The listing builds one solid part. Answer for the finished solid, in the listing's coordinates (mm). A direction names the side the tool comes from. Give positions to 0.01 mm unless a question says otherwise; leave off trailing zeros. Loops run counter-clockwise (first coordinate to the right, second up) from the corner with the lowest first, then second, coordinate; pieces in that order, holes last. Notation, with made-up numbers: (-4.75, 26) - (45.25, 26) arc R33 ccw to (45.25, 58) - close; hole circle Ø5 at (73.25, 60.25). An arc over 180 degrees is marked (long way). Write each question's results on one line, items separated by ' | '.
from build123d import *

# Parameters (mm, degrees)
SKETCH1_W           = 25.4
SKETCH1_H           = 25.4
SKETCH1_W_2         = 23
SKETCH1_H_2         = 23
BOSS_EXTRUDE1_DEPTH = 115
CUT_EXTRUDE1_START  = -24.2
SKETCH2_W           = 40.231781255
SKETCH2_H           = 27.281754711
CUT_EXTRUDE1_DEPTH  = 24.2
SKETCH5_R           = 1
SKETCH5_R_2         = 2.5
SKETCH5_R_3         = 1.25
CUT_EXTRUDE4_DEPTH  = 10
CUT_EXTRUDE2_REACH  = 142.365
SKETCH3_R           = 1.25
SKETCH3_R_2         = 1.05
SKETCH3_R_3         = 2.5
SKETCH6_R           = 1.6
SKETCH6_R_2         = 1.25
CUT_EXTRUDE5_DEPTH  = 8
SKETCH3_3_R         = 1.25
CUT_EXTRUDE9_DEPTH  = 141.364864582
SKETCH10_R          = 1.55
SKETCH10_R_2        = 1.25
SKETCH10_W          = 7.208576747
SKETCH10_H          = 12.490715562
SKETCH10_W_2        = 3.851256807
SKETCH10_H_2        = 11.057621271
CUT_EXTRUDE10_DEPTH = 5
FILLET1_R           = 3.5
SKETCH11_R          = 1.25
CUT_EXTRUDE11_DEPTH = 8


with BuildPart() as part:
    # Sketch1 → Boss-Extrude1 (new body)
    with BuildSketch(Plane.XY):
        with Locations((63.668417616, 21.669583611)):
            Rectangle(SKETCH1_W, SKETCH1_H)
        with Locations((63.668417616, 21.669583611)):
            Rectangle(SKETCH1_W_2, SKETCH1_H_2, mode=Mode.SUBTRACT)
    extrude(amount=BOSS_EXTRUDE1_DEPTH)

    # Sketch2 → Cut-Extrude1 (cut)
    with BuildSketch(Plane.ZY.offset(-50.968417616).offset(CUT_EXTRUDE1_START)):
        with Locations((94.884109373, 23.810460967)):
            Rectangle(SKETCH2_W, SKETCH2_H)
    extrude(amount=CUT_EXTRUDE1_DEPTH, mode=Mode.SUBTRACT)

    # Sketch5 → Cut-Extrude4 (cut)
    with BuildSketch(Plane(origin=(76.368417616, 0, 0), x_dir=(0, 0, -1), z_dir=(1, 0, 0))):
        with Locations((-102.757359313, 25.912224298)):
            Circle(SKETCH5_R)
        with Locations((-111.242640687, 25.912224298)):
            Circle(SKETCH5_R)
        with Locations((-111.242640687, 17.426942923)):
            Circle(SKETCH5_R)
        with Locations((-102.757359313, 17.426942923)):
            Circle(SKETCH5_R)
        with Locations((-107, 21.669583611)):
            Circle(SKETCH5_R_2)
        with Locations((-16.95, 29.737819564)):
            Circle(SKETCH5_R_3)
        with Locations((-75, 29.737819564)):
            Circle(SKETCH5_R_3)
        with Locations((-19.204163056, 23.117794927)):
            Circle(SKETCH5_R_3)
        with BuildLine():
            Line((-95.356264863, 19.604734734), (-95.356264863, 24.520728377))
            ThreePointArc((-95.356264863, 24.520728377), (-94.114846786, 25.762146454), (-92.87342871, 24.520728377))
            Line((-92.87342871, 24.520728377), (-92.87342871, 19.604734734))
            ThreePointArc((-92.87342871, 19.604734734), (-94.114846786, 18.363316658), (-95.356264863, 19.604734734))
        make_face()
    extrude(amount=-CUT_EXTRUDE4_DEPTH, mode=Mode.SUBTRACT)

    # Sketch3 → Cut-Extrude2 (cut, up to next)
    with BuildSketch(Plane.XZ.offset(-8.969583611), mode=Mode.PRIVATE) as cut_extrude2_sk1:
        with Locations(Location((54.918417616, 32, 0), (0, 0, 270))):
            Circle(SKETCH3_R)
    cut_extrude2_tool1 = extrude(cut_extrude2_sk1.sketch, amount=-CUT_EXTRUDE2_REACH, mode=Mode.PRIVATE) & part.part
    # Sketch3 → Cut-Extrude2 (cut, up to next)
    with BuildSketch(Plane.XZ.offset(-8.969583611), mode=Mode.PRIVATE) as cut_extrude2_sk2:
        with Locations(Location((54.918417616, 48, 0), (0, 0, 270))):
            Circle(SKETCH3_R)
    cut_extrude2_tool2 = extrude(cut_extrude2_sk2.sketch, amount=-CUT_EXTRUDE2_REACH, mode=Mode.PRIVATE) & part.part
    # Sketch3 → Cut-Extrude2 (cut, up to next)
    with BuildSketch(Plane.XZ.offset(-8.969583611), mode=Mode.PRIVATE) as cut_extrude2_sk3:
        with Locations(Location((56.439865007, 105.989791795, 0), (0, 0, 270))):
            Circle(SKETCH3_R_2)
    cut_extrude2_tool3 = extrude(cut_extrude2_sk3.sketch, amount=-CUT_EXTRUDE2_REACH, mode=Mode.PRIVATE) & part.part
    # Sketch3 → Cut-Extrude2 (cut, up to next)
    with BuildSketch(Plane.XZ.offset(-8.969583611), mode=Mode.PRIVATE) as cut_extrude2_sk4:
        with Locations(Location((62.439865007, 111.989791795, 0), (0, 0, 270))):
            Circle(SKETCH3_R_2)
    cut_extrude2_tool4 = extrude(cut_extrude2_sk4.sketch, amount=-CUT_EXTRUDE2_REACH, mode=Mode.PRIVATE) & part.part
    # Sketch3 → Cut-Extrude2 (cut, up to next)
    with BuildSketch(Plane.XZ.offset(-8.969583611), mode=Mode.PRIVATE) as cut_extrude2_sk5:
        with Locations(Location((68.439865007, 105.989791795, 0), (0, 0, 270))):
            Circle(SKETCH3_R_2)
    cut_extrude2_tool5 = extrude(cut_extrude2_sk5.sketch, amount=-CUT_EXTRUDE2_REACH, mode=Mode.PRIVATE) & part.part
    # Sketch3 → Cut-Extrude2 (cut, up to next)
    with BuildSketch(Plane.XZ.offset(-8.969583611), mode=Mode.PRIVATE) as cut_extrude2_sk6:
        with Locations(Location((62.439865007, 99.989791795, 0), (0, 0, 270))):
            Circle(SKETCH3_R_2)
    cut_extrude2_tool6 = extrude(cut_extrude2_sk6.sketch, amount=-CUT_EXTRUDE2_REACH, mode=Mode.PRIVATE) & part.part
    # Sketch3 → Cut-Extrude2 (cut, up to next)
    with BuildSketch(Plane.XZ.offset(-8.969583611), mode=Mode.PRIVATE) as cut_extrude2_sk7:
        with Locations(Location((62.439865007, 105.989791795, 0), (0, 0, 270))):
            Circle(SKETCH3_R_3)
    cut_extrude2_tool7 = extrude(cut_extrude2_sk7.sketch, amount=-CUT_EXTRUDE2_REACH, mode=Mode.PRIVATE) & part.part
    # Sketch3 → Cut-Extrude2 (cut, up to next)
    with BuildSketch(Plane.XZ.offset(-8.969583611), mode=Mode.PRIVATE) as cut_extrude2_sk8:
        with BuildLine():
            Line((65.785875381, 94.116283864), (70.188234194, 98.978147268))
            ThreePointArc((70.188234194, 98.978147268), (72.324899993, 99.084125699), (72.430878425, 96.947459901))
            Line((72.430878425, 96.947459901), (68.028519611, 92.085596497))
            ThreePointArc((68.028519611, 92.085596497), (65.891853813, 91.979618066), (65.785875381, 94.116283864))
        make_face()
    cut_extrude2_tool8 = extrude(cut_extrude2_sk8.sketch, amount=-CUT_EXTRUDE2_REACH, mode=Mode.PRIVATE) & part.part
    add(cut_extrude2_tool1.solids().sort_by_distance((54.918418, 8.969584, 32))[0], mode=Mode.SUBTRACT)
    add(cut_extrude2_tool2.solids().sort_by_distance((54.918418, 8.969584, 48))[0], mode=Mode.SUBTRACT)
    add(cut_extrude2_tool3.solids().sort_by_distance((56.439865, 8.969584, 105.989792))[0], mode=Mode.SUBTRACT)
    add(cut_extrude2_tool4.solids().sort_by_distance((62.439865, 8.969584, 111.989792))[0], mode=Mode.SUBTRACT)
    add(cut_extrude2_tool5.solids().sort_by_distance((68.439865, 8.969584, 105.989792))[0], mode=Mode.SUBTRACT)
    add(cut_extrude2_tool6.solids().sort_by_distance((62.439865, 8.969584, 99.989792))[0], mode=Mode.SUBTRACT)
    add(cut_extrude2_tool7.solids().sort_by_distance((62.439865, 8.969584, 105.989792))[0], mode=Mode.SUBTRACT)
    add(cut_extrude2_tool8.solids().sort_by_distance((69.108377, 8.969584, 95.531872))[0], mode=Mode.SUBTRACT)

    # Sketch6 → Cut-Extrude5 (cut)
    with BuildSketch(Plane(origin=(0, 8.969583611, 0), x_dir=(-1, 0, 0), z_dir=(0, -1, 0))):
        with Locations(Location((-70.405494882, -82.5, 0), (0, 0, 90))):
            Circle(SKETCH6_R)
        with Locations(Location((-56.074218123, -82.5, 0), (0, 0, 90))):
            Circle(SKETCH6_R)
        with Locations(Location((-61.706346911, -18.454172536, 0), (0, 0, 90))):
            Circle(SKETCH6_R_2)
    extrude(amount=-CUT_EXTRUDE5_DEPTH, mode=Mode.SUBTRACT)

    # Sketch3<3> → Cut-Extrude9 (cut, through all)
    with BuildSketch(Plane.XZ.offset(-8.969583611)):
        with Locations(Location((54.918417616, 32, 0), (0, 0, 270))):
            Circle(SKETCH3_3_R)
        with Locations(Location((54.918417616, 48, 0), (0, 0, 270))):
            Circle(SKETCH3_3_R)
    extrude(amount=-CUT_EXTRUDE9_DEPTH, mode=Mode.SUBTRACT)

    # Sketch10 → Cut-Extrude10 (cut)
    with BuildSketch(Plane(origin=(0, 34.369583611, 0), x_dir=(1, 0, 0), z_dir=(0, 1, 0))):
        with Locations(Location((63.038171916, -71.624774794, 0), (0, 0, 270))):
            Circle(SKETCH10_R)
        with Locations(Location((70.543887237, -71.685759742, 0), (0, 0, 270))):
            Circle(SKETCH10_R)
        with Locations(Location((61.706346911, -22.262070014, 0), (0, 0, 270))):
            Circle(SKETCH10_R_2)
        with Locations(Location((70.543887237, -13.635759742, 0), (0, 0, 270))):
            Circle(SKETCH10_R_2)
        with Locations((71.564129243, -52.463622479)):
            Rectangle(SKETCH10_W, SKETCH10_H)
        with Locations((52.89404602, -59.010132705)):
            Rectangle(SKETCH10_W_2, SKETCH10_H_2)
    extrude(amount=-CUT_EXTRUDE10_DEPTH, mode=Mode.SUBTRACT)

    # Fillet1
    fillet1_edges = [part.edges().sort_by_distance(p)[0] for p in [
        (67.959840869, 33.769583611, 58.70898026),
        (75.168417616, 33.769583611, 58.70898026),
    ]]
    fillet(fillet1_edges, radius=FILLET1_R)

    # Sketch11 → Cut-Extrude11 (cut)
    with BuildSketch(Plane.ZY.offset(-50.968417616)):
        with Locations(Location((22.262070014, 23.117794927, 0), (0, 0, 270))):
            Circle(SKETCH11_R)
    extrude(amount=-CUT_EXTRUDE11_DEPTH, mode=Mode.SUBTRACT)


solid = part.part
Item 1: A cutting plane is placed at B-B, the plane z = 48. Determine the outline of the cut face in (x, y).
Values found:
outline: (50.97, 8.97) - (53.67, 8.97) - (53.67, 10.17) - (52.17, 10.17) - (52.17, 33.17) - (53.67, 33.17) - (53.67, 34.37) - (50.97, 34.37) - close; (56.17, 8.97) - (76.37, 8.97) - (76.37, 34.37) - (75.17, 34.37) - (75.17, 10.17) - (56.17, 10.17) - close; (56.17, 33.17) - (67.96, 33.17) - (67.96, 34.37) - (56.17, 34.37) - close
Item 2: A cutting plane is placed at A-A, the plane z = 32. Determine the outline of the cut face in (x, y).
Values found:
outline: (50.97, 8.97) - (53.67, 8.97) - (53.67, 10.17) - (52.17, 10.17) - (52.17, 33.17) - (53.67, 33.17) - (53.67, 34.37) - (50.97, 34.37) - close; (56.17, 8.97) - (76.37, 8.97) - (76.37, 34.37) - (56.17, 34.37) - (56.17, 33.17) - (75.17, 33.17) - (75.17, 10.17) - (56.17, 10.17) - close
Item 3: For a pull along X with two mould halves and no side action, classify faces 4 (the face through (75.777, 28.518, 17.221)), 5 (the face through (70.26, 9.56, 94.55)) as released by +X, released by -X, zero draft, split by the parting line, or undercut.
Values found:
face 4: zero draft | face 5: undercut
Item 4: Flat-ended cylindrical pins translate along their axes: P1, Ø3, axis at x = 71.5, y = 31.5, coming from the -Z side; P2, Ø3, axis at x = 63.04, z = 71.62, coming from the +Y side; P3, Ø3, axis at y = 29, z = 91.5, coming from the -X side. Find the tip coordinate at first contact, or state that the pin passes through.
Values found:
P1: passes through | P2: stops at y = 10.17 | P3: stops at x = 75.17
Item 5: A cutting plane is placed at C-C, the plane z = 82.5. Determine the outline of the cut face in (x, y).
Values found:
outline: (50.97, 8.97) - (54.47, 8.97) - (54.47, 10.17) - (50.97, 10.17) - close; (57.67, 8.97) - (68.81, 8.97) - (68.81, 10.17) - (57.67, 10.17) - close; (72.01, 8.97) - (76.37, 8.97) - (76.37, 34.37) - (75.17, 34.37) - (75.17, 10.17) - (72.01, 10.17) - close
Item 6: Find the intervals of material crossed by line 1 along X through (y, z) = (13.25, 9); line 2 along Y through (x, z) = (72, 26.5); line 3 along Y through (x, z) = (76, 75), in increasing order. Write a range as [from, to].
Values found:
line 1: x = [50.97, 52.17], [75.17, 76.37] | line 2: y = [8.97, 10.17], [33.17, 34.37] | line 3: y = [8.97, 28.49], [30.99, 34.37]
Item 7: For faces 1 (the face through (69, 33.8, 57.7)), 2 (the face through (52, 32, 64.539)), 3 (the face through (75.777, 22.009, 18.627)), determine the directions among +Z, -Z, +X, -X, +Y, -Y from which every point of the face is accessible in a straight line to the end or side of a thin tool.
Values found:
face 1: +Y | face 2: -X, +Y | face 3: +X
